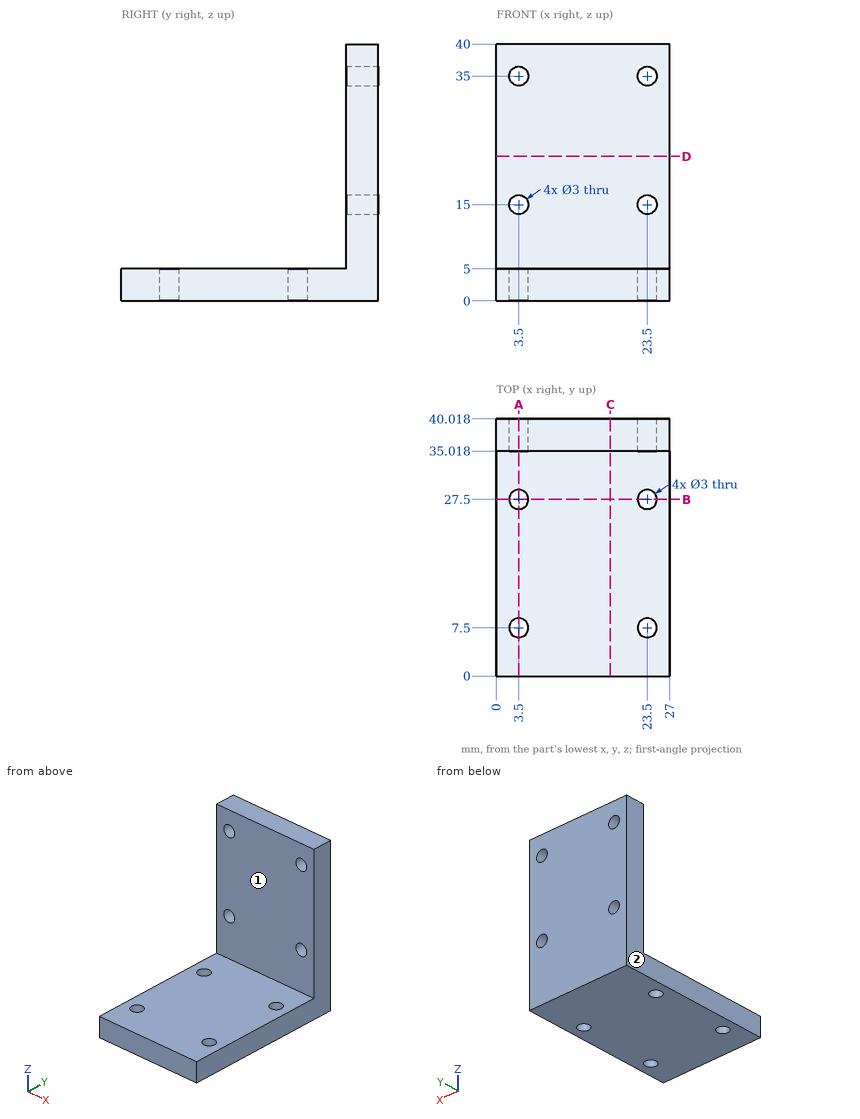
Can you work these out from the drawing? Everything is in mm from the part's minimum corner. A direction names the side the tool comes from. Coordinates: 2 decimals unless noted, no trailing zeros. Loops run counter-clockwise (first coordinate to the right, second up) from the corner with the lowest first, then second, coordinate; pieces in that order, holes last.
1) For pin 1 (2 mm diameter, centred on x = 9, z = 23, fed in from -Y); pin 2 (8 mm diameter, centred on x = 10.5, y = 16.5, fed in from +Z), each with a flat end and sliding along its axis, tell me the tip position at first contact or that it passes through.
2) Which directions (+Z, -Z, +X, -X, +Y, -Y) give clear straight access to the entire face, cutting with the end or side of a thin tool? Please do the marked faces 1 and 2.
3) Imagine slicing it at D-D on z = 22.5. List the corners of the cut face in (x, y) for me.
4) Imagine slicing it at C-C on x = 17.75. List the corners of the cut face in (y, z) for me.
5) Imagine slicing it at B-B on y = 27.5. List the corners of the cut face in (x, z) for me, plus the area to 3 significant figures.
6) Imagine slicing it at A-A on x = 3.5. List the corners of the cut face in (y, z) for me, plus the area to 3 significant figures.
7) I need wall thicknesses on probe 1 along Z at (x, y) = (3.5, 37.3); probe 2 along Y at (x, z) = (3.5, 1.6); probe 3 along Z at (x, y) = (23, 36). Which ranges of each line are inside material? Lowest first, please.
Completed:
1. pin 1: stops at y = 35.02
1. pin 2: stops at z = 5
2. face 1: +Z, +X, -X, -Y
2. face 2: +Z, -Z, -X, +Y, -Y
3. outline: (0, 35.02) - (27, 35.02) - (27, 40.02) - (0, 40.02) - close
4. outline: (0, 0) - (40.02, 0) - (40.02, 40) - (35.02, 40) - (35.02, 5) - (0, 5) - close
5. outline: (0, 0) - (2, 0) - (2, 5) - (0, 5) - close; (5, 0) - (22, 0) - (22, 5) - (5, 5) - close; (25, 0) - (27, 0) - (27, 5) - (25, 5) - close
5. area: 105 mm2
6. outline: (0, 0) - (6, 0) - (6, 5) - (0, 5) - close; (9, 0) - (26, 0) - (26, 5) - (9, 5) - close; (29, 0) - (40.02, 0) - (40.02, 13.5) - (35.02, 13.5) - (35.02, 5) - (29, 5) - close; (35.02, 16.5) - (40.02, 16.5) - (40.02, 33.5) - (35.02, 33.5) - close; (35.02, 36.5) - (40.02, 36.5) - (40.02, 40) - (35.02, 40) - close
6. area: 315 mm2
7. probe 1: z = 0 to 13.5, 16.5 to 33.5, 36.5 to 40
7. probe 2: y = 0 to 6, 9 to 26, 29 to 40.02
7. probe 3: z = 0 to 13.59, 16.41 to 33.59, 36.41 to 40
